For this review, take the finished solid that the model builds, in its own axes (mm). Face numbers are marked on the shaded views. A direction names the side the tool comes from. Round coordinates to 2 decimals unless told otherwise and drop trailing zeros. Loops run counter-clockwise (first coordinate to the right, second up) from the corner with the lowest first, then second, coordinate; pieces in that order, holes last.
1) Take a section at C-C (y = 1). State the section outline as (x, z) points, then the cut area to 3 significant figures.
2) Take a section at D-D (z = 2.5). State the section outline as (x, y) points, then the cut area to 3 significant figures.
3) Take a section at B-B (y = -3.25). State the section outline as (x, z) points, then the cut area to 3 significant figures.
4) Take a section at A-A (x = -26). State the section outline as (y, z) points.
5) Wall thickness on L1, parallel to X at y = 0.7, z = 12.5; L2, parallel to Z at x = -4, y = -10.75; L3, parallel to Y at x = -18, z = -10: over which ranges is each line inside the solid? List them lowest first.
6) Mouldability with a two-part tool opening along X and no side actions: class the marked faces 4 and 5 as pulls with the +X half, pulls with the -X half, needs draft (parallel to the pull), parting line crosses it, or undercut.
7) Tool access review of the marked faces 1, 2 and 3: name each direction out of +Z, -Z, +X, -X, +Y, -Y from which nothing blocks a thin tool from reaching the whole face with its end or side.
8) Insertion check: pin 1 (6.5 mm diameter, centred on x = -26.5, z = 1.5, fed in from +Y); pin 2 (1.8 mm diameter, centred on x = 26, z = 12.5, fed in from -Y); pin 3 (4 mm diameter, centred on x = 23, z = -10.5, fed in from +Y); pin 4 (2.5 mm diameter, centred on x = 16.5, y = 3.5, fed in from +Z). Each pin has a flat end and moves straight along its axis. Give the tip position at first contact, or say it passes through.
```python
from build123d import *

# Parameters (mm, degrees)
SKETCH1_W          = 58
SKETCH1_H          = 31
CIRCUIT_DEPTH      = 1.6
SKETCH2_W          = 24.2
SKETCH2_H          = 16
ESP_PCB_DEPTH      = 1
SKETCH3_W          = 15.2
SKETCH3_H          = 12
ESP_CHIP_DEPTH     = 2.5
SKETCH4_W          = 5
SKETCH4_H          = 7
PCB_HOLES_DEPTH    = 2.5
SKETCH5_R          = 1.5
CUT_EXTRUDE1_DEPTH = 34.068111528
SKETCH6_W          = 7
SKETCH6_H          = 2.5
USB_DEPTH          = 1
SKETCH7_W          = 38
SKETCH7_H          = 2.5
PINS_DEPTH         = 20


with BuildPart() as part:
    # Sketch1 → CIRCUIT (new body)
    with BuildSketch(Plane(origin=(0, 0, 0), x_dir=(1, 0, 0), z_dir=(0, 1, 0))):
        Rectangle(SKETCH1_W, SKETCH1_H)
    extrude(amount=CIRCUIT_DEPTH)

    # Sketch2 → ESP_PCB (add)
    with BuildSketch(Plane(origin=(0, 1.6, 0), x_dir=(1, 0, 0), z_dir=(0, 1, 0))):
        with Locations((16.9, 0)):
            Rectangle(SKETCH2_W, SKETCH2_H)
    extrude(amount=ESP_PCB_DEPTH)

    # Sketch3 → ESP_CHIP (add)
    with BuildSketch(Plane(origin=(0, 2.6, 0), x_dir=(1, 0, 0), z_dir=(0, 1, 0))):
        with Locations((13.4, 0)):
            Rectangle(SKETCH3_W, SKETCH3_H)
    extrude(amount=ESP_CHIP_DEPTH)

    # Sketch4 → PCB_HOLES (add)
    with BuildSketch(Plane(origin=(0, 1.6, 0), x_dir=(1, 0, 0), z_dir=(0, 1, 0))):
        with Locations((-26.5, 0)):
            Rectangle(SKETCH4_W, SKETCH4_H)
    extrude(amount=PCB_HOLES_DEPTH)

    # Sketch5 → Cut-Extrude1 (cut, through all)
    with BuildSketch(Plane(origin=(0, 1.6, 0), x_dir=(1, 0, 0), z_dir=(0, 1, 0))):
        with Locations(Location((-26, 12.5, 0), (0, 0, 270))):
            Circle(SKETCH5_R)
        with Locations(Location((-26, -12.5, 0), (0, 0, 270))):
            Circle(SKETCH5_R)
        with Locations(Location((26, 12.5, 0), (0, 0, 270))):
            Circle(SKETCH5_R)
        with Locations(Location((26, -12.5, 0), (0, 0, 270))):
            Circle(SKETCH5_R)
    extrude(amount=-CUT_EXTRUDE1_DEPTH, mode=Mode.SUBTRACT)

    # Sketch6 → USB (add)
    with BuildSketch(Plane.ZY.offset(29)):
        with Locations((0, 2.85)):
            Rectangle(SKETCH6_W, SKETCH6_H)
    extrude(amount=USB_DEPTH)

    # Sketch7 → PINS (add)
    with BuildSketch(Plane.XZ):
        with Locations((0, 14.25)):
            Rectangle(SKETCH7_W, SKETCH7_H)
        with Locations((0, -14.25)):
            Rectangle(SKETCH7_W, SKETCH7_H)
    extrude(amount=PINS_DEPTH)


solid = part.part
```
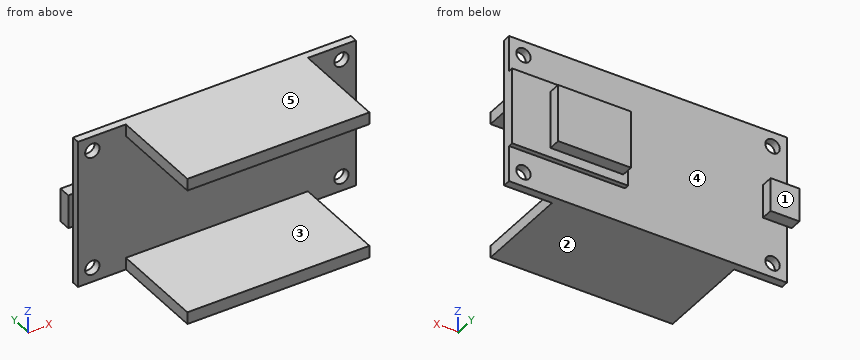
Response:
1. outline: (-29, -15.5) - (29, -15.5) - (29, 15.5) - (-29, 15.5) - close; hole circle Ø3 at (-26, -12.5); hole circle Ø3 at (-26, 12.5); hole circle Ø3 at (26, -12.5); hole circle Ø3 at (26, 12.5)
1. area: 1,770 mm2
2. outline: (-30, 1.6) - (-29, 1.6) - (-29, 0) - (29, 0) - (29, 2.6) - (21, 2.6) - (21, 5.1) - (5.8, 5.1) - (5.8, 2.6) - (4.8, 2.6) - (4.8, 1.6) - (-24, 1.6) - (-24, 4.1) - (-30, 4.1) - close
2. area: 170 mm2
3. outline: (-19, -15.5) - (19, -15.5) - (19, -13) - (-19, -13) - close; (-19, 13) - (19, 13) - (19, 15.5) - (-19, 15.5) - close
3. area: 190 mm2
4. outline: (0, -15.5) - (1.6, -15.5) - (1.6, -14) - (0, -14) - close; (0, -11) - (1.6, -11) - (1.6, -3.5) - (4.1, -3.5) - (4.1, 3.5) - (1.6, 3.5) - (1.6, 11) - (0, 11) - close; (0, 14) - (1.6, 14) - (1.6, 15.5) - (0, 15.5) - close
5. L1: x = -29 to -27.5, -24.5 to 24.5, 27.5 to 29
5. L2: z = -15.5 to -13, 13 to 15.5
5. L3: y = 0 to 1.6
6. face 4: undercut
6. face 5: needs draft
7. face 1: +Z, -Z, -X, +Y
7. face 2: -Z, +X, -X, +Y, -Y
7. face 3: +X, -X, -Y
8. pin 1: stops at y = 4.1
8. pin 2: passes through
8. pin 3: stops at y = 1.6
8. pin 4: stops at z = 8
